For this review, take the finished solid that the model builds, in its own axes (mm). Round coordinates to 2 decimals unless told otherwise and drop trailing zeros. Write each loop counter-clockwise with the first axis right and the second up, starting at its lowest first coordinate (ties: lowest second). Pieces come first, ordered by that corner, then holes. Notation, with made-up numbers: (2.5, 68.25) -> (18.5, 68.25) arc R21 ccw to (18.5, 80.25) -> close; hole circle Ø3 at (35, 14.25). An arc over 180 degrees is marked (long way). Answer in a Markdown table with one row per item.
from build123d import *

# Parameters (mm, degrees)
SKETCH2_W           = 359
SKETCH2_H           = 210
BOSS_EXTRUDE1_DEPTH = 5.25
SKETCH3_W           = 349.5
SKETCH3_H           = 197.5
CUT_EXTRUDE1_DEPTH  = 0.1
BOSS_EXTRUDE2_DEPTH = 1
SKETCH5_W           = 226.5
SKETCH5_H           = 41
BOSS_EXTRUDE3_DEPTH = 0.25


with BuildPart() as part:
    # Sketch2 → Boss-Extrude1 (new body)
    with BuildSketch(Plane.XY):
        Rectangle(SKETCH2_W, SKETCH2_H)
    extrude(amount=BOSS_EXTRUDE1_DEPTH)

    # Sketch3 → Cut-Extrude1 (cut)
    with BuildSketch(Plane.XY.offset(5.25)):
        with Locations((0.75, 0.25)):
            Rectangle(SKETCH3_W, SKETCH3_H)
    extrude(amount=-CUT_EXTRUDE1_DEPTH, mode=Mode.SUBTRACT)

    # Sketch4 → Boss-Extrude2 (add)
    with BuildSketch(Plane(origin=(0, 0, 0), x_dir=(-1, 0, 0), z_dir=(0, 0, -1))):
        Polygon((-71.8, -69), (-71.8, -70), (-74.3, -70), (-74.3, -66), (-71.8, -66), (-71.8, -67), (-50.8, -67), (-50.8, -66), (-48.3, -66), (-48.3, -70), (-50.8, -70), (-50.8, -69), align=None)
    extrude(amount=BOSS_EXTRUDE2_DEPTH)

    # Sketch5 → Boss-Extrude3 (add)
    with BuildSketch(Plane(origin=(0, 0, 0), x_dir=(-1, 0, 0), z_dir=(0, 0, -1))):
        with Locations((-0.25, -84.5)):
            Rectangle(SKETCH5_W, SKETCH5_H)
    extrude(amount=BOSS_EXTRUDE3_DEPTH)


solid = part.part
1) Consider section B-B on y = 90. State the section outline as (x, z) points.
Solved:
| item | result |
|---|---|
| outline | (-179.5, 0) -> (179.5, 0) -> (179.5, 5.25) -> (175.5, 5.25) -> (175.5, 5.15) -> (-174, 5.15) -> (-174, 5.25) -> (-179.5, 5.25) -> close |
2) For line 1 (Z direction, x = -11.5, y = -94); line 2 (Z direction, x = 34, y = 7.5), list the stretches that pass through material, from the lowest coordinate up. Write a range as [from, to].
Solved:
| item | result |
|---|---|
| line 1 | [-0.25, 5.15] |
| line 2 | [0, 5.15] |
3) Consider section A-A on x = 86. State the section outline as (y, z) points.
Solved:
| item | result |
|---|---|
| outline | (-105, -0.25) -> (-64, -0.25) -> (-64, 0) -> (105, 0) -> (105, 5.25) -> (99, 5.25) -> (99, 5.15) -> (-98.5, 5.15) -> (-98.5, 5.25) -> (-105, 5.25) -> close |
4) Clearance check with flat-ended pins moving along their axes: pin 1 Ø2 at (x, y) = (42, 57) entering from +Z; pin 2 Ø1.5 at (x, y) = (-134, -65) entering from -Z; pin 3 Ø0.8 at (y, z) = (-69.5, -0.5) entering from +X. State where each tip first meets the part, or that it passes through.
Solved:
| item | result |
|---|---|
| pin 1 | z = 5.15 |
| pin 2 | z = 0 |
| pin 3 | x = 113.5 |
5) Consider section C-C on x = 147. State the section outline as (y, z) points, then the cut area to 3 significant figures.
Solved:
| item | result |
|---|---|
| outline | (-105, 0) -> (105, 0) -> (105, 5.25) -> (99, 5.25) -> (99, 5.15) -> (-98.5, 5.15) -> (-98.5, 5.25) -> (-105, 5.25) -> close |
| area | 1,080 mm² |
